from build123d import *

# Parameters (mm, degrees)
ESQUISSE1_R                  = 11
ESQUISSE1_R_2                = 3.5
BOSS_EXTRU_1_DEPTH           = 0.4
ESQUISSE2_W                  = 1
ESQUISSE2_H                  = 4
ENL_V_MAT_EXTRU_1_DEPTH      = 16.561490931
R_P_TITION_CIRCULAIRE1_COUNT = 18


with BuildPart() as part:
    # Esquisse1 → Boss.-Extru.1 (new body)
    with BuildSketch(Plane.XY):
        Circle(ESQUISSE1_R)
        Circle(ESQUISSE1_R_2, mode=Mode.SUBTRACT)
    extrude(amount=BOSS_EXTRU_1_DEPTH)

    # Esquisse2 → Enlèv. mat.-Extru.1 (cut, symmetric)
    with BuildSketch(Plane.XY.offset(0.4)):
        with Locations((0, 7.25)):
            Rectangle(ESQUISSE2_W, ESQUISSE2_H)
    enl_v_mat_extru_1 = extrude(amount=ENL_V_MAT_EXTRU_1_DEPTH, both=True, mode=Mode.SUBTRACT)

    # Répétition circulaire1: Enlèv. mat.-Extru.1 ×18 about axis
    r_p_tition_circulaire1_axis = Axis((0, 0, 0), (0, 0, 1))
    for i in range(1, R_P_TITION_CIRCULAIRE1_COUNT):
        add(enl_v_mat_extru_1.rotate(r_p_tition_circulaire1_axis, i * 360 / R_P_TITION_CIRCULAIRE1_COUNT), mode=Mode.SUBTRACT)


solid = part.part
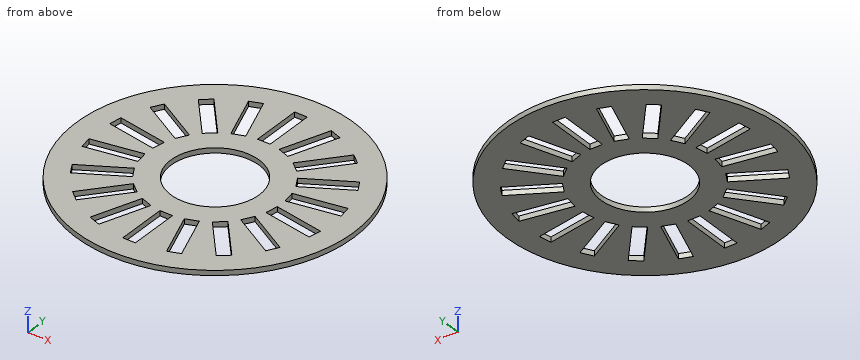
Verification items for the finished model (mm, model axes). Coordinates: 2 decimals unless noted, no trailing zeros. Order: outer loops, then holes, each group sorted by start corner. A loop starts at its lowest first (then second) coordinate and runs counter-clockwise, first axis right, second up. Notation, with made-up numbers: M 88,-0.5 L 136,-0.5 A29 cw 136,33.5 Z; hole C 53.25,77.25 d11. An arc over 180 degrees is marked long. Return JSON: item names as keys, results as strings.
1) Cross-section at B-B, the plane y = 0. Record the boundary of the cut face in (x, z), and give its area (3 significant figures).
Answer list:
{"outline": "M -11,0 L -3.5,0 L -3.5,0.4 L -11,0.4 Z; M 3.5,0 L 11,0 L 11,0.4 L 3.5,0.4 Z", "area": "6.00 mm2"}
2) Cross-section at D-D, the plane x = 7. Record the boundary of the cut face in (y, z).
Answer list:
{"outline": "M -8.49,0 L -4.62,0 L -4.62,0.4 L -8.49,0.4 Z; M -3.46,0 L -1.74,0 L -1.74,0.4 L -3.46,0.4 Z; M -0.73,0 L 0.73,0 L 0.73,0.4 L -0.73,0.4 Z; M 1.74,0 L 3.46,0 L 3.46,0.4 L 1.74,0.4 Z; M 4.62,0 L 8.49,0 L 8.49,0.4 L 4.62,0.4 Z"}
3) Cross-section at C-C, the plane y = -8.25. Record the boundary of the cut face in (x, z), and give its area (3 significant figures).
Answer list:
{"outline": "M -7.28,0 L -3.53,0 L -3.53,0.4 L -7.28,0.4 Z; M -2.47,0 L -0.5,0 L -0.5,0.4 L -2.47,0.4 Z; M 0.5,0 L 2.47,0 L 2.47,0.4 L 0.5,0.4 Z; M 3.53,0 L 7.28,0 L 7.28,0.4 L 3.53,0.4 Z", "area": "4.57 mm2"}
4) Thickness scan on L1, parallel to Y at x = 0, z = 0.2; L2, parallel to X at y = 4.5, z = 0.2; L3, parallel to X at y = -8, z = 0.3. Record the ranges inside material, lowest first. Write a range as [from, to].
Answer list:
{"L1": "[-11, -9.25], [-5.25, -3.5], [3.5, 5.25], [9.25, 11]", "L2": "[-10.04, -8.08], [-6.79, -4.43], [-3.12, 3.12], [4.43, 6.79], [8.08, 10.04]", "L3": "[-7.55, -3.44], [-2.38, -0.5], [0.5, 2.38], [3.44, 7.55]"}
5) Gauge pin test, flat end, axial feed: pin 1 (4 mm diameter, centred on x = 0, y = 0, fed in from +Z) (3 decimals). Record the tip position at first contact, or that the pin passes through.
Answer list:
{"pin 1": "through"}
6) Cross-section at A-A, the plane x = 0. Record the boundary of the cut face in (y, z).
Answer list:
{"outline": "M -11,0 L -9.25,0 L -9.25,0.4 L -11,0.4 Z; M -5.25,0 L -3.5,0 L -3.5,0.4 L -5.25,0.4 Z; M 3.5,0 L 5.25,0 L 5.25,0.4 L 3.5,0.4 Z; M 9.25,0 L 11,0 L 11,0.4 L 9.25,0.4 Z"}
